Part model, mm, in its own coordinate system. A direction names the side the tool comes from. Give positions to 0.01 mm unless a question says otherwise; leave off trailing zeros. Write each loop counter-clockwise with the first axis right and the second up, starting at its lowest first coordinate (ties: lowest second). Pieces come first, ordered by that corner, then holes.
from build123d import *

# Parameters (mm, degrees)
SKETCH2_R          = 14
CUT_EXTRUDE1_DEPTH = 30


with BuildPart() as part:
    # Sketch1 → Revolve1 (revolve)
    with BuildSketch(Plane.XY, mode=Mode.PRIVATE) as revolve1_sk:
        with BuildLine():
            Line((0, -20), (18, -20))
            Line((18, -20), (18, 10))
            Line((18, 10), (24, 10))
            ThreePointArc((24, 10), (26.121320344, 10.878679656), (27, 13))
            Line((27, 13), (27, 17))
            ThreePointArc((27, 17), (26.121320344, 19.121320344), (24, 20))
            Line((24, 20), (0, 20))
            Line((0, 20), (0, -20))
        make_face()
    revolve(revolve1_sk.sketch.rotate(Axis((0, 20, 0), (0, -1, 0)), 180), axis=Axis((0, 20, 0), (0, -1, 0)))

    # Sketch2 → Cut-Extrude1 (cut)
    with BuildSketch(Plane.XZ.offset(20)):
        Circle(SKETCH2_R)
    extrude(amount=-CUT_EXTRUDE1_DEPTH, mode=Mode.SUBTRACT)


solid = part.part
1) Saw through at C-C (y = 14.5). Write the cut outline in (x, z), and give its area (3 significant figures).
Check result:
outline: circle Ø54 at (0, 0)
area: 2,290 mm2
2) Saw through at A-A (x = 0). Write the cut outline in (y, z), and give its area (3 significant figures).
Check result:
outline: (-20, -18) - (10, -18) - (10, -24) arc R3 ccw to (13, -27) - (17, -27) arc R3 ccw to (20, -24) - (20, 24) arc R3 ccw to (17, 27) - (13, 27) arc R3 ccw to (10, 24) - (10, 18) - (-20, 18) - (-20, 14) - (10, 14) - (10, -14) - (-20, -14) - close
area: 772 mm2
3) Flat gauge pins, fed straight in: P1, Ø10, axis at x = 14, y = 5.5, coming from the -Z side; P2, Ø6, axis at x = -19.5, z = -19.5, coming from the -Y side; P3, Ø8, axis at y = -5.5, z = 14, coming from the -X side. Where does each tip first touch, or does it go through?
Check result:
P1: stops at z = -21.96
P2: stops at y = 10.06
P3: stops at x = -14.97
4) Saw through at B-B (z = 0). Write the cut outline in (x, y), and give its area (3 significant figures).
Check result:
outline: (-27, 13) arc R3 ccw to (-24, 10) - (-18, 10) - (-18, -20) - (-14, -20) - (-14, 10) - (14, 10) - (14, -20) - (18, -20) - (18, 10) - (24, 10) arc R3 ccw to (27, 13) - (27, 17) arc R3 ccw to (24, 20) - (-24, 20) arc R3 ccw to (-27, 17) - close
area: 772 mm2
5) Drill centre lines: L1, parallel to Z at x = 0, y = -2; L2, parallel to Z at x = 12, y = 9; L3, parallel to Y at x = -1.5, z = -12. Where is each one in solid material? Low to high.
Check result:
L1: z = -18 to -14, 14 to 18
L2: z = -13.42 to -7.21, 7.21 to 13.42
L3: y = 10 to 20
6) Mould opens along X. For faces 1 (the flat face through (0, 10, 0)), 2 (the flat face through (9, -20, 11)), 3 (the cylindrical face through (13.267, -4.79, -12.165)) say: +X half, -X half, draft (parallel to the pull), parting line (faces both ways), or undercut.
Check result:
face 1: undercut
face 2: draft
face 3: parting line
7) Saw through at D-D (y = -4.5). Write the cut outline in (x, z).
Check result:
outline: circle Ø36 at (0, 0); hole circle Ø28 at (0, 0)
8) 3-axis set-ups, long thin cutter, end or side, ignore diameter. For faces 4 (the flat face through (0, 20, 0)), 5 (the flat face through (3, 10, -18)): which of +Z, -Z, +X, -X, +Y, -Y reach the whole face in a straight line?
Check result:
face 4: +Z, -Z, +X, -X, +Y
face 5: -Y
